```python
from build123d import *

# Parameters (mm, degrees)
F2_R     = 10
F3_DEPTH = 100
F4_SIZE2 = 2
F4_SIZE  = 5
F5_R     = 1.5
F6_DEPTH = 50
F9_R     = 5
F10_R    = 5


# Not quite as in the source:
# - two fillets or chamfers of one size are made in one step


with BuildPart() as f3:
    # F2 (on Top) → F3 (new body)
    with BuildSketch(Plane.XY):
        Circle(F2_R)
    extrude(amount=F3_DEPTH)

    # F4
    f4_edges = [f3.edges().sort_by_distance(p)[0] for p in [
        (-10, 0, 0),
    ]]
    f4_side = f3.faces().sort_by_distance((-10, 0, 50))[0]
    chamfer(f4_edges, length=F4_SIZE, length2=F4_SIZE2, reference=f4_side)

    # F5 (on face) → F6 (cut)
    with BuildSketch(Plane.XY.offset(100)):
        Circle(F5_R)
    extrude(amount=-F6_DEPTH, mode=Mode.SUBTRACT)

    # F7 (on Front) → F8 (revolve, cut)
    with BuildSketch(Plane.XZ):
        with BuildLine():
            Line((13.1810711939, 79.0897459622), (13.1810711939, 97.5897459622))
            ThreePointArc((13.1810711939, 97.5897459622), (6.9807422323, 88.3397459622), (13.1810711939, 79.0897459622))
        make_face()
    revolve(axis=Axis((0, 0, 50), (0, 0, -1)), mode=Mode.SUBTRACT)

    # F9
    f9_edges = [f3.edges().sort_by_distance(p)[0] for p in [
        (-10, 0, 81.179492),
    ]]
    fillet(f9_edges, radius=F9_R)

    # F10
    f10_edges = [f3.edges().sort_by_distance(p)[0] for p in [
        (-10, 0, 5),
        (-10, 0, 95.5),
    ]]
    fillet(f10_edges, radius=F10_R)


solid = f3.part
```
Design review of the part built by this model. Coordinates are the model's own, in mm. A direction names the side the tool comes from. Coordinates: 2 decimals unless noted, no trailing zeros. Order: outer loops, then holes, each group sorted by start corner. A loop starts at its lowest first (then second) coordinate and runs counter-clockwise, first axis right, second up. Notation, with made-up numbers: M 15,-39 L 36,-39 A17 ccw 36,-9 Z; hole C 43.25,-35.5 d3. An arc over 180 degrees is marked long. Answer as a JSON object with one key per item and string values. Group by question number.
1) Add section A-A, the plane z = 67.5. Write out the cut boundary in (x, y), then the cut area to 3 significant figures.
2) Add section B-B, the plane z = 45. Write out the cut boundary in (x, y), then the cut area to 3 significant figures.
3) For pin 1 (1.5 mm diameter, centred on x = -1.5, z = 86.5, fed in from -Y); pin 2 (4 mm diameter, centred on x = -6.5, z = 59, fed in from -Y); pin 3 (4 mm diameter, centred on x = -3, z = 41, fed in from +Y), all flat-tipped, find the tip position at first contact; note any pin that passes through.
4) Mouldability with a two-part tool opening along Y and no side actions: class faces 1 (the flat face through (2, 0, 100)), 2 (the cylindrical face through (-2.17, -9.76, 42.13)), 3 (the cylindrical face through (-1.5, 0.07, 75.35)) as pulls with the +Y half, pulls with the -Y half, needs draft (parallel to the pull), parting line crosses it, or undercut.
5) Tool access review of faces 4 (the cylindrical face through (9.54, 3, 98.66)), 5 (the flat face through (0, 0, 50)): name each direction out of +Z, -Z, +X, -X, +Y, -Y from which nothing blocks a thin tool from reaching the whole face with its end or side.
6) Wall thickness on L1, parallel to Y at x = 0, z = 62.5; L2, parallel to Z at x = 7, y = 6; L3, parallel to Y at x = 6, z = 76.5: over which ranges is each line inside the solid? List them lowest first.
Computed values:
{
 "1": {"outline": "C 0,0 d20; hole C 0,0 d3", "area": "307 mm^2"},
 "2": {"outline": "C 0,0 d20", "area": "314 mm^2"},
 "3": {"pin 1": "stops at y = -7.21", "pin 2": "stops at y = -8.93", "pin 3": "stops at y = 9.95"},
 "4": {"face 1": "needs draft", "face 2": "parting line crosses it", "face 3": "undercut"},
 "5": {"face 4": "+Z, -Z", "face 5": "+Z"},
 "6": {"L1": "y = -10 to -1.5, 1.5 to 10", "L2": "z = 3.05 to 82, 94.68 to 100", "L3": "y = -8 to 8"}
}
